```python
from build123d import *

# Parameters (mm, degrees)
SKETCH_1_R      = 2
SKETCH_1_R_2    = 2.5
SKETCH_1_R_3    = 6
SKETCH_1_W      = 400
SKETCH_1_H      = 200
EXTRUDE_1_DEPTH = 3


with BuildPart() as part:
    # 草图1 → 凸台-拉伸1 (new body)
    with BuildSketch(Plane(origin=(0, 0, 0), x_dir=(1, 0, 0), z_dir=(0, 1, 0))):
        with BuildLine():
            Line((2, 0), (648, 0))
            ThreePointArc((648, 0), (649.414213562, 0.585786438), (650, 2))
            Line((650, 2), (650, 348))
            ThreePointArc((650, 348), (649.414213562, 349.414213562), (648, 350))
            Line((648, 350), (2, 350))
            ThreePointArc((2, 350), (0.585786438, 349.414213562), (0, 348))
            Line((0, 348), (0, 2))
            ThreePointArc((0, 2), (0.585786438, 0.585786438), (2, 0))
        make_face()
        with Locations(Location((13, 13, 0), (0, 0, 270))):
            Circle(SKETCH_1_R, mode=Mode.SUBTRACT)
        with Locations(Location((637, 13, 0), (0, 0, 270))):
            Circle(SKETCH_1_R, mode=Mode.SUBTRACT)
        with Locations(Location((13, 337, 0), (0, 0, 270))):
            Circle(SKETCH_1_R, mode=Mode.SUBTRACT)
        with Locations(Location((637, 337, 0), (0, 0, 270))):
            Circle(SKETCH_1_R, mode=Mode.SUBTRACT)
        with Locations(Location((475, 50.49256144, 0), (0, 0, 270))):
            Circle(SKETCH_1_R_2, mode=Mode.SUBTRACT)
        with Locations(Location((175, 50, 0), (0, 0, 270))):
            Circle(SKETCH_1_R_2, mode=Mode.SUBTRACT)
        with Locations(Location((25, 60, 0), (0, 0, 270))):
            Circle(SKETCH_1_R_3, mode=Mode.SUBTRACT)
        with Locations((325, 200)):
            Rectangle(SKETCH_1_W, SKETCH_1_H, mode=Mode.SUBTRACT)
    extrude(amount=-EXTRUDE_1_DEPTH)


solid = part.part
```
Verification items for the finished model (mm, model axes). Give positions to 0.01 mm unless a question says otherwise; leave off trailing zeros. Loops run counter-clockwise (first coordinate to the right, second up) from the corner with the lowest first, then second, coordinate; pieces in that order, holes last.
1. Thickness scan on line 1 (Z direction, x = 637, y = -2.3); line 2 (Z direction, x = 475, y = -2.3); line 3 (Z direction, x = 334.5, y = -2.2). Record the ranges inside material, lowest first.
2. Section check C-C, the plane y = -0.65. Count the separate pieces of the cut face and the enclosed holes in it, then the cut area to 3 significant figures.
3. Section check A-A, the plane z = -255. Enter the section's corners in (x, y), then the cut area to 3 significant figures.
4. Mould release check, pull along X, two halves, no side actions. Record for faces 1 (the cylindrical face through (25, -1, -66)), 2 (the flat face through (320.5, -3, -99.7)): released by +X, released by -X, zero draft, split by the parting line, or undercut.
5. Section check B-B, the plane x = 464. Enter the section's corners in (y, z).
Geometry says:
1. line 1: z = -350 to -339, -335 to -15, -11 to 0
1. line 2: z = -350 to -300, -100 to -52.99, -47.99 to 0
1. line 3: z = -350 to -300, -100 to 0
2. separate pieces: 1
2. enclosed holes: 8
2. area: 147,000 mm2
3. outline: (0, -3) - (125, -3) - (125, 0) - (0, 0) - close; (525, -3) - (650, -3) - (650, 0) - (525, 0) - close
3. area: 750 mm2
4. face 1: undercut
4. face 2: zero draft
5. outline: (-3, -350) - (0, -350) - (0, -300) - (-3, -300) - close; (-3, -100) - (0, -100) - (0, 0) - (-3, 0) - close
